Here's how the part is built. I have some questions about the finished solid (model axes, mm). Face numbers are marked on the shaded views. A direction names the side the tool comes from. Round coordinates to 2 decimals unless told otherwise and drop trailing zeros. Order: outer loops, then holes, each group sorted by start corner. A loop starts at its lowest first (then second) coordinate and runs counter-clockwise, first axis right, second up.
```python
from build123d import *

# Parameters (mm, degrees)
EXTRUDE_1_DEPTH     = 46
SKETCH_2_R          = 1.5
SKETCH_2_R_2        = 5
CUT_EXTRUDE_1_DEPTH = 56
CUT_EXTRUDE_2_DEPTH = 56


with BuildPart() as part:
    # 草图1 → 凸台-拉伸1 (new body)
    with BuildSketch(Plane.XY):
        Polygon((0, 0), (30, 0), (30, 3), (3, 3), (3, 38), (0, 38), align=None)
    extrude(amount=EXTRUDE_1_DEPTH)

    # 草图2 → 切除-拉伸1 (cut)
    with BuildSketch(Plane(origin=(3, 0, 0), x_dir=(0, 0, -1), z_dir=(1, 0, 0))):
        with Locations(Location((-39.5, 31, 0), (0, 0, 90))):
            Circle(SKETCH_2_R)
        with Locations(Location((-39.5, 13, 0), (0, 0, 90))):
            Circle(SKETCH_2_R)
        with Locations(Location((-6.5, 31, 0), (0, 0, 90))):
            Circle(SKETCH_2_R)
        with Locations(Location((-6.5, 13, 0), (0, 0, 90))):
            Circle(SKETCH_2_R)
        with Locations(Location((-31, 22, 0), (0, 0, 90))):
            Circle(SKETCH_2_R_2)
        with Locations(Location((-15, 22, 0), (0, 0, 90))):
            Circle(SKETCH_2_R_2)
    extrude(amount=-CUT_EXTRUDE_1_DEPTH, mode=Mode.SUBTRACT)

    # 草图3 → 切除-拉伸2 (cut)
    with BuildSketch(Plane(origin=(0, 3, 0), x_dir=(1, 0, 0), z_dir=(0, 1, 0))):
        with BuildLine():
            Line((9.5, -5), (23.5, -5))
            ThreePointArc((23.5, -5), (25.5, -7), (23.5, -9))
            Line((23.5, -9), (9.5, -9))
            ThreePointArc((9.5, -9), (7.5, -7), (9.5, -5))
        make_face()
        with BuildLine():
            Line((9.5, -37), (23.5, -37))
            ThreePointArc((23.5, -37), (25.5, -39), (23.5, -41))
            Line((23.5, -41), (9.5, -41))
            ThreePointArc((9.5, -41), (7.5, -39), (9.5, -37))
        make_face()
    extrude(amount=-CUT_EXTRUDE_2_DEPTH, mode=Mode.SUBTRACT)


solid = part.part
```
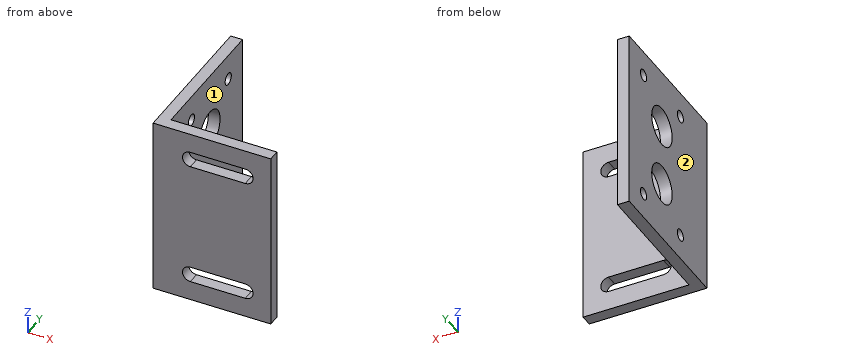
1) I'm going to push flat-ended pins straight in: pin 1 (1.8 mm diameter, centred on y = 13, z = 6.5, fed in from +X); pin 2 (5 mm diameter, centred on y = 13, z = 39.5, fed in from +X); pin 3 (4 mm diameter, centred on x = 22.5, z = 22.5, fed in from +Y). Where does each tip first touch, or does it pass through?
2) If we section it at C-C (x = 18.5): Write out the boundary of the cut face in (y, z), plus the area to 3 significant figures.
3) If we section it at B-B (z = 19): Write out the boundary of the cut face in (x, y).
4) If we section it at A-A (y = 31): Write out the boundary of the cut face in (x, z), plus the area to 3 significant figures.
5) If we section it at D-D (z = 6.5): Write out the boundary of the cut face in (x, y).
6) For the marked faces 1 and 2, which set-ups out of +Z, -Z, +X, -X, +Y, -Y let a thin tool reach every point of the face, with its end or its side?
7) I need wall thicknesses on line 1 (Z direction, x = 0.65, y = 13); line 2 (Z direction, x = 1.5, y = 22); line 3 (X direction, y = 31.5, z = 25.5). Which ranges of each line are inside material? Lowest first, please.
Solutions:
1. pin 1: passes through
1. pin 2: stops at x = 3
1. pin 3: stops at y = 3
2. outline: (0, 0) - (3, 0) - (3, 5) - (0, 5) - close; (0, 9) - (3, 9) - (3, 37) - (0, 37) - close; (0, 41) - (3, 41) - (3, 46) - (0, 46) - close
2. area: 114 mm2
3. outline: (0, 0) - (30, 0) - (30, 3) - (3, 3) - (3, 19) - (0, 19) - close; (0, 25) - (3, 25) - (3, 38) - (0, 38) - close
4. outline: (0, 0) - (3, 0) - (3, 5) - (0, 5) - close; (0, 8) - (3, 8) - (3, 38) - (0, 38) - close; (0, 41) - (3, 41) - (3, 46) - (0, 46) - close
4. area: 120 mm2
5. outline: (0, 0) - (7.56, 0) - (7.56, 3) - (3, 3) - (3, 11.5) - (0, 11.5) - close; (0, 14.5) - (3, 14.5) - (3, 29.5) - (0, 29.5) - close; (0, 32.5) - (3, 32.5) - (3, 38) - (0, 38) - close; (25.44, 0) - (30, 0) - (30, 3) - (25.44, 3) - close
6. face 1: +Z, -Z, +X, +Y
6. face 2: +Z, -Z, -X, +Y, -Y
7. line 1: z = 0 to 5, 8 to 38, 41 to 46
7. line 2: z = 0 to 10, 20 to 26, 36 to 46
7. line 3: x = 0 to 3
